Could you check a few things on this model? Use its own coordinates, in mm. A direction names the side the tool comes from. Round coordinates to 2 decimals unless told otherwise and drop trailing zeros. Write each loop counter-clockwise with the first axis right and the second up, starting at its lowest first coordinate (ties: lowest second). Pieces come first, ordered by that corner, then holes. Notation, with made-up numbers: (-32, 47) -> (-10, 47) arc R4 ccw to (-10, 53) -> close; hole circle Ø8 at (36.25, -4.5). An arc over 180 degrees is marked (long way). Answer in a Markdown table with one row per item.
from build123d import *

# Parameters (mm, degrees)
SKETCH_1_R          = 4.5
SKETCH_1_R_2        = 1.25
EXTRUDE_1_DEPTH     = 8.5
EXTRUDE_2_DEPTH     = 12
CHAMFER_1_SIZE      = 2.5
SKETCH_2_R          = 8
CUT_EXTRUDE_1_DEPTH = 6
FILLET_1_R          = 2
FILLET_2_R          = 0.5


with BuildPart() as part:
    # Sketch 1 → Extrude 1 (new body)
    with BuildSketch(Plane(origin=(0, 0, 0), x_dir=(1, 0, 0), z_dir=(0, 1, 0))):
        with BuildLine():
            ThreePointArc((-14.641038215, 21), (-18.101933598, 18.101933598), (-21, 14.641038215))
            Line((-21, 14.641038215), (-21, -14.641038215))
            ThreePointArc((-21, -14.641038215), (-18.101933598, -18.101933598), (-14.641038215, -21))
            Line((-14.641038215, -21), (14.641038215, -21))
            ThreePointArc((14.641038215, -21), (18.101933598, -18.101933598), (21, -14.641038215))
            Line((21, -14.641038215), (21, 14.641038215))
            ThreePointArc((21, 14.641038215), (18.101933598, 18.101933598), (14.641038215, 21))
            Line((14.641038215, 21), (-14.641038215, 21))
        make_face()
        Circle(SKETCH_1_R, mode=Mode.SUBTRACT)
        with Locations((-15.5, 15.5)):
            Circle(SKETCH_1_R_2, mode=Mode.SUBTRACT)
        with Locations((15.5, 15.5)):
            Circle(SKETCH_1_R_2, mode=Mode.SUBTRACT)
        with Locations((15.5, -15.5)):
            Circle(SKETCH_1_R_2, mode=Mode.SUBTRACT)
        with Locations((-15.5, -15.5)):
            Circle(SKETCH_1_R_2, mode=Mode.SUBTRACT)
    extrude(amount=EXTRUDE_1_DEPTH)

    # Sketch 1_4 → Extrude 2 (add)
    with BuildSketch(Plane(origin=(0, 0, 0), x_dir=(1, 0, 0), z_dir=(0, 1, 0))):
        with BuildLine():
            ThreePointArc((21, -14.641038215), (18.101933598, -18.101933598), (14.641038215, -21))
            Line((14.641038215, -21), (17.2, -21))
            Line((17.2, -21), (21, -17.2))
            Line((21, -17.2), (21, -14.641038215))
        make_face()
        with BuildLine():
            ThreePointArc((-14.641038215, -21), (-18.101933598, -18.101933598), (-21, -14.641038215))
            Line((-21, -14.641038215), (-21, -17.2))
            Line((-21, -17.2), (-17.2, -21))
            Line((-17.2, -21), (-14.641038215, -21))
        make_face()
        with BuildLine():
            Line((-17.2, 21), (-21, 17.2))
            Line((-21, 17.2), (-21, 14.641038215))
            ThreePointArc((-21, 14.641038215), (-18.101933598, 18.101933598), (-14.641038215, 21))
            Line((-14.641038215, 21), (-17.2, 21))
        make_face()
        with BuildLine():
            Line((17.2, 21), (14.641038215, 21))
            ThreePointArc((14.641038215, 21), (18.101933598, 18.101933598), (21, 14.641038215))
            Line((21, 14.641038215), (21, 17.2))
            Line((21, 17.2), (17.2, 21))
        make_face()
    extrude(amount=EXTRUDE_2_DEPTH)

    # Chamfer 1
    chamfer_1_edges = [part.edges().sort_by_distance(p)[0] for p in [
        (-16.75, 0, 15.5),
        (14.25, 0, 15.5),
        (14.25, 0, -15.5),
        (-16.75, 0, -15.5),
    ]]
    chamfer(chamfer_1_edges, length=CHAMFER_1_SIZE)

    # Sketch 2 → Cut-Extrude 1 (cut)
    with BuildSketch(Plane(origin=(0, 8.5, 0), x_dir=(1, 0, 0), z_dir=(0, 1, 0))):
        Circle(SKETCH_2_R)
    extrude(amount=-CUT_EXTRUDE_1_DEPTH, mode=Mode.SUBTRACT)

    # Fillet 1
    fillet_1_edges = [part.edges().sort_by_distance(p)[0] for p in [
        (17.2, 6, 21),
        (21, 6, 17.2),
        (-21, 6, 17.2),
        (-17.2, 6, 21),
        (-17.2, 6, -21),
        (-21, 6, -17.2),
        (21, 6, -17.2),
        (17.2, 6, -21),
    ]]
    fillet(fillet_1_edges, radius=FILLET_1_R)

    # Fillet 2
    fillet_2_edges = [part.edges().sort_by_distance(p)[0] for p in [
        (21, 0, 0),
        (0, 0, 21),
        (-19.1, 0, 19.1),
        (-21, 0, 0),
        (-19.1, 0, -19.1),
        (0, 0, -21),
        (19.1, 0, -19.1),
        (19.1, 0, 19.1),
        (20.847759065, 0, -17.13693974),
        (17.13693974, 0, -20.847759065),
        (-17.13693974, 0, -20.847759065),
        (-20.847759065, 0, -17.13693974),
        (-20.847759065, 0, 17.13693974),
        (-17.13693974, 0, 20.847759065),
        (17.13693974, 0, 20.847759065),
        (20.847759065, 0, 17.13693974),
    ]]
    fillet(fillet_2_edges, radius=FILLET_2_R)


solid = part.part
1) Please list where these lines run through material, in increasing order: line 1 (X direction, y = 6.55, z = 15.5); line 2 (X direction, y = 8, z = 0).
Findings:
| item | result |
|---|---|
| line 1 | x = -21 to -16.75, -14.25 to 14.25, 16.75 to 21 |
| line 2 | x = -21 to -8, 8 to 21 |
2) Imagine slicing it at B-B, the plane z = 0. Please give me the cut outline in (x, y), plus the area to 3 significant figures.
Findings:
| item | result |
|---|---|
| outline | (-21, 0.5) arc R0.5 ccw to (-20.5, 0) -> (-4.5, 0) -> (-4.5, 2.5) -> (-8, 2.5) -> (-8, 8.5) -> (-21, 8.5) -> close; (4.5, 0) -> (20.5, 0) arc R0.5 ccw to (21, 0.5) -> (21, 8.5) -> (8, 8.5) -> (8, 2.5) -> (4.5, 2.5) -> close |
| area | 238 mm^2 |
3) For pin 1 (8 mm diameter, centred on x = -1, z = 2, fed in from +Y); pin 2 (21 mm diameter, centred on x = -9, z = -7, fed in from +Y); pin 3 (4 mm diameter, centred on x = 15.5, z = -15.5, fed in from -Y); pin 4 (1.5 mm diameter, centred on x = -15.5, z = 15.5, fed in from -Y), each with a flat end and sliding along its axis, tell me the tip position at first contact or that it passes through.
Findings:
| item | result |
|---|---|
| pin 1 | stops at y = 2.5 |
| pin 2 | stops at y = 8.5 |
| pin 3 | stops at y = 1.75 |
| pin 4 | passes through |
4) Thinking about a two-plate mould opening in X: for faces 3 (the face through (19, 12, -18)), 4 (the face through (-16.87, 2.38, 15.44)), 5 (the face through (19.1, 6.2, -19.1)), which applies, +X half, -X half, draft (parallel to the pull), parting line (faces both ways), or undercut?
Findings:
| item | result |
|---|---|
| face 3 | draft |
| face 4 | undercut |
| face 5 | +X half |
5) Imagine slicing it at D-D, the plane x = 15.5. Please give me the cut outline in (y, z), plus the area to 3 significant figures.
Findings:
| item | result |
|---|---|
| outline | (0, -20.5) arc R0.5 ccw to (0.5, -21) -> (12, -21) -> (12, -20.37) -> (8.5, -20.37) -> (8.5, -16.75) -> (2.5, -16.75) -> (0, -19.25) -> close; (0, -11.75) -> (2.5, -14.25) -> (8.5, -14.25) -> (8.5, 14.25) -> (2.5, 14.25) -> (0, 11.75) -> close; (0, 19.25) -> (2.5, 16.75) -> (8.5, 16.75) -> (8.5, 20.37) -> (12, 20.37) -> (12, 21) -> (0.5, 21) arc R0.5 ccw to (0, 20.5) -> close |
| area | 306 mm^2 |
6) Imagine slicing it at A-A, the plane x = 0. Please give me the cut outline in (y, z).
Findings:
| item | result |
|---|---|
| outline | (0, -20.5) arc R0.5 ccw to (0.5, -21) -> (8.5, -21) -> (8.5, -8) -> (2.5, -8) -> (2.5, -4.5) -> (0, -4.5) -> close; (0, 4.5) -> (2.5, 4.5) -> (2.5, 8) -> (8.5, 8) -> (8.5, 21) -> (0.5, 21) arc R0.5 ccw to (0, 20.5) -> close |
7) For faces 1 (the face through (17.147, 6.33, -20.844)), 2 (the face through (-1.73, 5.54, 7.81)), which set-ups out of +Z, -Z, +X, -X, +Y, -Y let a thin tool reach every point of the face, with its end or its side?
Findings:
| item | result |
|---|---|
| face 1 | -Z, +X, +Y, -Y |
| face 2 | +Y |
8) Imagine slicing it at C-C, the plane y = 9.25. Please give me the cut outline in (x, z), plus the area to 3 significant figures.
Findings:
| item | result |
|---|---|
| outline | (-21, -16.37) arc R2 ccw to (-20.41, -17.79) -> (-17.79, -20.41) arc R2 ccw to (-16.37, -21) -> (-14.64, -21) arc R25.6 cw to (-21, -14.64) -> close; (-21, 14.64) arc R25.6 cw to (-14.64, 21) -> (-16.37, 21) arc R2 ccw to (-17.79, 20.41) -> (-20.41, 17.79) arc R2 ccw to (-21, 16.37) -> close; (14.64, -21) -> (16.37, -21) arc R2 ccw to (17.79, -20.41) -> (20.41, -17.79) arc R2 ccw to (21, -16.37) -> (21, -14.64) arc R25.6 cw to start; (14.64, 21) arc R25.6 cw to (21, 14.64) -> (21, 16.37) arc R2 ccw to (20.41, 17.79) -> (17.79, 20.41) arc R2 ccw to (16.37, 21) -> close |
| area | 41.7 mm^2 |
